Print and shaded views of the part. All mm, measured from the part's lowest x, y and z. Give positions to 0.01 mm unless a question says otherwise; leave off trailing zeros. Order: outer loops, then holes, each group sorted by start corner. A loop starts at its lowest first (then second) coordinate and runs counter-clockwise, first axis right, second up. Notation, with made-up numbers: (6.5, -11) - (40.5, -11) arc R4 ccw to (40.5, -4) - close; hole circle Ø6 at (89, 27.25). An arc over 180 degrees is marked (long way). Answer in a Markdown table with one row per item.
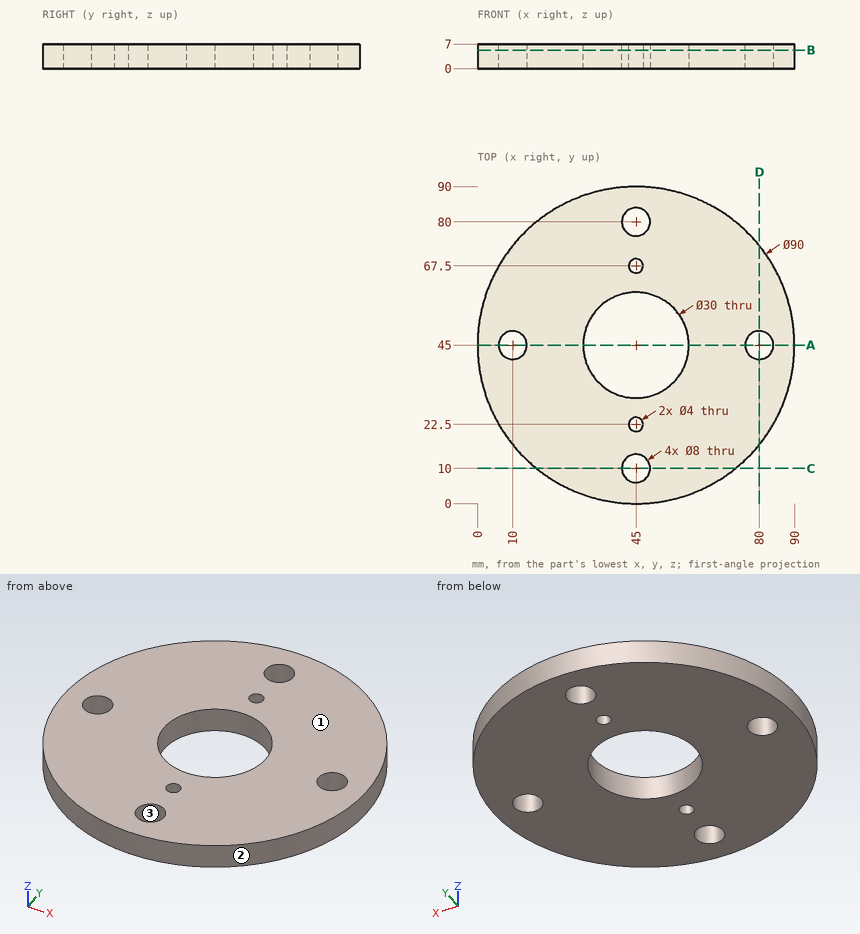
1. Cut at B-B on z = 5.25. Write the cut outline in (x, y).
Check result:
| item | result |
|---|---|
| outline | circle Ø90 at (45, 45); hole circle Ø8 at (10, 45); hole circle Ø30 at (45, 45); hole circle Ø8 at (45, 10); hole circle Ø8 at (45, 80); hole circle Ø4 at (45, 22.5); hole circle Ø4 at (45, 67.5); hole circle Ø8 at (80, 45) |
2. Probe line 1 (Y direction, x = 45, z = 5.25); line 2 (Y direction, x = 48, z = 4.25); line 3 (X direction, y = 36, z = 0.75). List the from-to ranges inside material, lowest first.
Check result:
| item | result |
|---|---|
| line 1 | y = 0 to 6, 14 to 20.5, 24.5 to 30, 60 to 65.5, 69.5 to 76, 84 to 90 |
| line 2 | y = 0.1 to 7.35, 12.65 to 30.3, 59.7 to 77.35, 82.65 to 89.9 |
| line 3 | x = 0.91 to 33, 57 to 89.09 |
3. Two-plate mould, pull along Y, no slides. Class the marked faces 1, 2 and 3: +Y half, -Y half, draft (parallel to the pull), parting line (faces both ways), or undercut.
Check result:
| item | result |
|---|---|
| face 1 | draft |
| face 2 | parting line |
| face 3 | undercut |
4. Cut at A-A on y = 45. Write the cut outline in (x, z), and give its area (3 significant figures).
Check result:
| item | result |
|---|---|
| outline | (0, 0) - (6, 0) - (6, 7) - (0, 7) - close; (14, 0) - (30, 0) - (30, 7) - (14, 7) - close; (60, 0) - (76, 0) - (76, 7) - (60, 7) - close; (84, 0) - (90, 0) - (90, 7) - (84, 7) - close |
| area | 308 mm² |
5. Drop a flat-ended pin along its axis: P1, Ø7, axis at x = 10, y = 45, coming from the +Z side. Give the stop position or say it passes through.
Check result:
| item | result |
|---|---|
| P1 | passes through |
6. Cut at C-C on y = 10. Write the cut outline in (x, z), and give its area (3 significant figures).
Check result:
| item | result |
|---|---|
| outline | (16.72, 0) - (41, 0) - (41, 7) - (16.72, 7) - close; (49, 0) - (73.28, 0) - (73.28, 7) - (49, 7) - close |
| area | 340 mm² |
